Source: CAD feature listing. Evaluate the final solid. Frame: model axes, mm. A direction names the side the tool comes from. Round coordinates to 2 decimals unless told otherwise and drop trailing zeros. Loops run counter-clockwise (first coordinate to the right, second up) from the corner with the lowest first, then second, coordinate; pieces in that order, holes last. Notation, with made-up numbers: (-17, 18) -> (12, 18) arc R35 ccw to (12, 53) -> close; hole circle Ø5 at (7, 5). An arc over 180 degrees is marked (long way). Return JSON: item names as keys, results as strings. Group by question number.
```python
from build123d import *

# Parameters (mm, degrees)
SKETCH1_W               = 72
SKETCH1_H               = 60
BOSS_EXTRUDE1_DEPTH     = 5
SKETCH2_W               = 5
SKETCH2_H               = 60
BOSS_EXTRUDE2_DEPTH     = 70
SKETCH3_W               = 5
SKETCH3_H               = 60
BOSS_EXTRUDE3_DEPTH     = 70
BOSS_EXTRUDE4_DEPTH     = 60
CHAMFER1_SIZE           = 42
CHAMFER1_SIZE_2         = 35.242184509
CHAMFER2_SIZE           = 15.000718891
CHAMFER2_SIZE_2         = 50
SKETCH12_W              = 20.2
SKETCH12_H              = 20.2
CUT_EXTRUDE8_DEPTH      = 67
CUT_EXTRUDE1_DEPTH      = 117.978630527
CUT_EXTRUDE1_DEPTH_BACK = 117.978630527
SKETCH5_R               = 12.5
SKETCH6_R               = 1.65
CUT_EXTRUDE2_DEPTH      = 121.037494142
SKETCH7_R               = 4
CUT_EXTRUDE4_DEPTH      = 117.978630527
CUT_EXTRUDE5_DEPTH      = 105.748460609
CUT_EXTRUDE5_DEPTH_BACK = 105.748460609
SKETCH8_R               = 2.65
CUT_EXTRUDE6_DEPTH      = 121.037494142
CUT_EXTRUDE6_DEPTH_BACK = 121.037494142
SKETCH9_R               = 2.65
FILLET1_R               = 5
SKETCH10_R              = 2.65
CUT_EXTRUDE7_DEPTH      = 10


with BuildPart() as part:
    # Sketch1 → Boss-Extrude1 (new body)
    with BuildSketch(Plane(origin=(0, 0, 0), x_dir=(1, 0, 0), z_dir=(0, 1, 0))):
        with Locations((36, 30)):
            Rectangle(SKETCH1_W, SKETCH1_H)
    extrude(amount=BOSS_EXTRUDE1_DEPTH)

    # Sketch2 → Boss-Extrude2 (add)
    with BuildSketch(Plane(origin=(0, 5, 0), x_dir=(1, 0, 0), z_dir=(0, 1, 0))):
        with Locations((2.5, 30)):
            Rectangle(SKETCH2_W, SKETCH2_H)
    extrude(amount=BOSS_EXTRUDE2_DEPTH)

    # Sketch3 → Boss-Extrude3 (add)
    with BuildSketch(Plane(origin=(0, 5, 0), x_dir=(1, 0, 0), z_dir=(0, 1, 0))):
        with Locations((27.7, 30)):
            Rectangle(SKETCH3_W, SKETCH3_H)
    extrude(amount=BOSS_EXTRUDE3_DEPTH)

    # Sketch11 → Boss-Extrude4 (add)
    with BuildSketch(Plane(origin=(0, 0, -60), x_dir=(-1, 0, 0), z_dir=(0, 0, -1))):
        Polygon((-25.2, 25), (-15.1, 35.1), (-5, 25), (-5, 75), (-25.2, 75), align=None)
    extrude(amount=-BOSS_EXTRUDE4_DEPTH)

    # Chamfer1
    # the kernel refuses this chamfer: 42, 35.242184509 mm, written as the material it adds along each edge
    with BuildSketch(Plane(origin=(30.2, 5, -60), x_dir=(0.9996889667359942, -0.02493932209023436, 0), z_dir=(0, 0, 1))) as chamfer1_piece_1_section:
        Polygon((CHAMFER1_SIZE * 0.999688966736, CHAMFER1_SIZE * 0.0249393220902), (-CHAMFER1_SIZE_2 * 0.0249393220905, CHAMFER1_SIZE_2 * 0.999688966749), (0, 0), align=None)
    chamfer1_piece_1 = extrude(amount=60, mode=Mode.PRIVATE)
    chamfer1_piece_1 = split(chamfer1_piece_1, bisect_by=Plane(origin=(72, 16.573415306, -30), z_dir=(-1, 0, 0)), keep=Keep.TOP, mode=Mode.PRIVATE)
    add(chamfer1_piece_1)

    # Chamfer2
    # the kernel refuses this chamfer: 50, 15.000718891 mm, written as the material it takes off along each edge
    with BuildSketch(Plane(origin=(159.997065138, 75, -60), x_dir=(0, 0.12207157319780576, 0.9925213000318999), z_dir=(-1, 0, 0))) as chamfer2_piece_1:
        Polygon((CHAMFER2_SIZE * 0.99252130002, -CHAMFER2_SIZE * 0.122071573196), (-CHAMFER2_SIZE_2 * 0.122071573198, -CHAMFER2_SIZE_2 * 0.992521300032), (0, 0), align=None)
    extrude(amount=289.794130277, mode=Mode.SUBTRACT)
    with BuildSketch(Plane(origin=(159.997065138, 75, 0), x_dir=(0, 0.12207157319780576, -0.9925213000318999), z_dir=(-1, 0, 0))) as chamfer2_piece_2:
        Polygon((CHAMFER2_SIZE * 0.99252130002, CHAMFER2_SIZE * 0.122071573196), (-CHAMFER2_SIZE_2 * 0.122071573198, CHAMFER2_SIZE_2 * 0.992521300032), (0, 0), align=None)
    extrude(amount=289.794130277, mode=Mode.SUBTRACT)

    # Sketch12 → Cut-Extrude8 (cut)
    with BuildSketch(Plane(origin=(0, 75, 0), x_dir=(1, 0, 0), z_dir=(0, 1, 0))):
        with Locations((15.1, 30)):
            Rectangle(SKETCH12_W, SKETCH12_H)
    extrude(amount=-CUT_EXTRUDE8_DEPTH, mode=Mode.SUBTRACT)

    # Sketch5 → Cut-Extrude1 (cut, two sides: drawn at the far end of the back side and taken through both)
    with BuildSketch(Plane(origin=(0, 5, 0), x_dir=(1, 0, 0), z_dir=(0, 1, 0)).offset(-CUT_EXTRUDE1_DEPTH_BACK)):
        with Locations(Location((51, 30, 0), (0, 0, 270))):
            Circle(SKETCH5_R)
    extrude(amount=CUT_EXTRUDE1_DEPTH + CUT_EXTRUDE1_DEPTH_BACK, mode=Mode.SUBTRACT)

    # Sketch6 → Cut-Extrude2 (cut, through all)
    with BuildSketch(Plane.XZ):
        with Locations(Location((66.5, -14.5, 0), (0, 0, 270))):
            Circle(SKETCH6_R)
        with Locations(Location((66.5, -45.5, 0), (0, 0, 270))):
            Circle(SKETCH6_R)
        with Locations(Location((35.5, -45.5, 0), (0, 0, 270))):
            Circle(SKETCH6_R)
        with Locations(Location((35.5, -14.5, 0), (0, 0, 270))):
            Circle(SKETCH6_R)
    extrude(amount=-CUT_EXTRUDE2_DEPTH, mode=Mode.SUBTRACT)

    # Sketch7 → Cut-Extrude4 (cut, through all)
    with BuildSketch(Plane(origin=(0, 5, 0), x_dir=(1, 0, 0), z_dir=(0, 1, 0))):
        with Locations((66.5, 45.5)):
            Circle(SKETCH7_R)
        with Locations((66.5, 14.5)):
            Circle(SKETCH7_R)
        with Locations((35.5, 14.5)):
            Circle(SKETCH7_R)
        with Locations((35.5, 45.5)):
            Circle(SKETCH7_R)
    extrude(amount=CUT_EXTRUDE4_DEPTH, mode=Mode.SUBTRACT)

    # Sketch8 → Cut-Extrude5 (cut, two sides: drawn at the far end of the back side and taken through both)
    with BuildSketch(Plane(origin=(30.2, 0, 0), x_dir=(0, 0, -1), z_dir=(1, 0, 0)).offset(-CUT_EXTRUDE5_DEPTH_BACK)):
        with Locations((30, 65)):
            Circle(SKETCH8_R)
    extrude(amount=CUT_EXTRUDE5_DEPTH + CUT_EXTRUDE5_DEPTH_BACK, mode=Mode.SUBTRACT)

    # Sketch9 → Cut-Extrude6 (cut, two sides: drawn at the far end of the back side and taken through both)
    with BuildSketch(Plane.XZ.offset(-CUT_EXTRUDE6_DEPTH_BACK)):
        with Locations(Location((15, -30, 0), (0, 0, 270))):
            Circle(SKETCH9_R)
    extrude(amount=CUT_EXTRUDE6_DEPTH + CUT_EXTRUDE6_DEPTH_BACK, mode=Mode.SUBTRACT)

    # Fillet1
    fillet1_edges = [part.edges().sort_by_distance(p)[0] for p in [
        (72, 2.583909963, -60),
        (72, 2.583909963, 0),
    ]]
    fillet(fillet1_edges, radius=FILLET1_R)

    # Sketch10 → Cut-Extrude7 (cut)
    with BuildSketch(Plane.ZY):
        with Locations((-30, 15)):
            Circle(SKETCH10_R)
    extrude(amount=-CUT_EXTRUDE7_DEPTH, mode=Mode.SUBTRACT)


solid = part.part
```
(1) Cut plane A-A (y = 15). Return loops of the section in (x, z), and give its area (3 significant figures).
(2) Ray query, line 1 (Y direction, x = 2.6, z = -30); line 2 (X direction, y = 7.25, z = -45.5); line 3 (Z direction, x = 35.5, y = 24.5). Return the intervals inside material, ascending.
(3) Cut plane B-B (z = -29). Count the separate pieces of the cut face and the enclosed holes in it, and give its area (3 significant figures).
(4) Cut plane C-C (y = 27.5). Return loops of the section in (x, z).
(5) Cut plane D-D (x = 43). Return loops of the section in (y, z).
(6) Set-up query: faces 1 (the face through (30.2, 57, -30)), 2 (the face through (10, 5, -30)), 3 (the face through (15, 50, -40.1)). Return all of +Z, -Z, +X, -X, +Y, -Y with unobstructed straight access to the full face (end or side cutting, diameter ignored); none if empty.
(7) Mould query, pull axis Z, two halves, no side actions, for faces 4 (the face through (64.9, 2.5, -45.1)), 5 (the face through (20.2, 30, -50.2)), 6 (the face through (70, 4, -1)). Classes: released by +Z, released by -Z, zero draft, split by the parting line, or undercut.
(8) Pin query (flat end, axial travel): pin 1 (5 mm diameter, centred on x = 20.5, y = 67.5, fed in from -Z); pin 2 (10 mm diameter, centred on y = 53.5, z = -19, fed in from +X); pin 3 (2.5 mm diameter, centred on x = 65, z = -46, fed in from +Y); pin 4 (3 mm diameter, centred on x = 66.5, z = -45.5, fed in from +Y). Return the tip coordinate at first contact, or that it passes through.
Answers follow:
{
 "1": {"outline": "(0, -60) -> (5, -60) -> (5, -32.65) -> (0, -32.65) -> close; (0, -27.35) -> (5, -27.35) -> (5, 0) -> (0, 0) -> close; (25.2, -60) -> (60.28, -60) -> (60.28, -38.37) arc R12.5 cw (long way) to (60.28, -21.63) -> (60.28, 0) -> (25.2, 0) -> close; hole circle Ø8 at (35.5, -45.5); hole circle Ø8 at (35.5, -14.5)", "area": "1,820 mm^2"},
 "2": {"line 1": "0 to 12.35, 17.65 to 62.35, 67.65 to 75", "line 2": "0 to 5, 25.2 to 31.5, 39.5 to 62.5", "line 3": "-60 to -49.5, -41.5 to -18.5, -10.5 to 0"},
 "3": {"separate pieces": "6", "enclosed holes": "0", "area": "1,130 mm^2"},
 "4": {"outline": "(0, -59.25) -> (7.5, -59.25) -> (7.5, -40.1) -> (5, -40.1) -> (5, -19.9) -> (7.5, -19.9) -> (7.5, -0.75) -> (0, -0.75) -> close; (22.7, -59.25) -> (45.39, -59.25) -> (45.39, -41.17) arc R12.5 cw to (45.39, -18.83) -> (45.39, -0.75) -> (22.7, -0.75) -> (22.7, -19.9) -> (25.2, -19.9) -> (25.2, -40.1) -> (22.7, -40.1) -> close; hole circle Ø8 at (35.5, -45.5); hole circle Ø8 at (35.5, -14.5)"},
 "5": {"outline": "(0, -60) -> (25, -60) -> (29.5, -58.65) -> (29.5, -39.6) -> (0, -39.6) -> close; (0, -20.4) -> (29.5, -20.4) -> (29.5, -1.35) -> (25, 0) -> (0, 0) -> close"},
 "6": {"face 1": "+Z, -Z, +X, +Y", "face 2": "+Z, -Z", "face 3": "+Y"},
 "7": {"face 4": "undercut", "face 5": "zero draft", "face 6": "released by +Z"},
 "8": {"pin 1": "z = -48", "pin 2": "x = 30.2", "pin 3": "y = 5", "pin 4": "through"}
}
